Verification items for the finished model (mm, model axes). A direction names the side the tool comes from. Round coordinates to 2 decimals unless told otherwise and drop trailing zeros. Loops run counter-clockwise (first coordinate to the right, second up) from the corner with the lowest first, then second, coordinate; pieces in that order, holes last. Notation, with made-up numbers: (-10.5, -39) - (43.5, -39) arc R29 cw to (43.5, -14) - close; hole circle Ø10 at (-4, 33). An arc over 180 degrees is marked (long way). Use a Markdown table: item, result. Add a question column.
```python
from build123d import *

# Parameters (mm, degrees)
CUT_EXTRUDE_START        = -35
CUT_EXTRUDE_1_DEPTH      = 35
CUT_EXTRUDE_2_DEPTH      = 185.932420089
CUT_EXTRUDE_2_DEPTH_BACK = 185.932420089
SKETCH_4_R               = 7
SKETCH_4_R_2             = 10
SKETCH_5_W               = 35
SKETCH_5_H               = 14
CUT_EXTRUDE_3_DEPTH      = 4
CHAMFER_1_SIZE           = 2


with BuildPart() as part:
    # Эскиз2 → Повернуть1 (revolve)
    with BuildSketch(Plane.XY):
        Polygon((0, 0), (0, 20), (60, 20), (60, 30), (110, 30), (110, 24), (180, 24), (180, 0), align=None)
    revolve(axis=Axis((180, 0, 0), (-1, 0, 0)))

    # Эскиз3 → Вырез-Вытянуть1 (cut)
    with BuildSketch(Plane.ZY.offset(CUT_EXTRUDE_START)):
        with BuildLine():
            Line((-16, 12), (16, 12))
            ThreePointArc((16, 12), (0, 20), (-16, 12))
        make_face()
    extrude(amount=CUT_EXTRUDE_1_DEPTH, mode=Mode.SUBTRACT)

    # Эскиз4 → Вырез-Вытянуть2 (cut, two sides: drawn at the far end of the back side and taken through both)
    with BuildSketch(Plane(origin=(0, 0, 0), x_dir=(1, 0, 0), z_dir=(0, 1, 0)).offset(-CUT_EXTRUDE_2_DEPTH_BACK)):
        with Locations(Location((17.5, 0, 0), (0, 0, 270))):
            Circle(SKETCH_4_R)
        with Locations(Location((85, 0, 0), (0, 0, 270))):
            Circle(SKETCH_4_R_2)
    extrude(amount=CUT_EXTRUDE_2_DEPTH + CUT_EXTRUDE_2_DEPTH_BACK, mode=Mode.SUBTRACT)

    # Эскиз5 → Вырез-Вытянуть3 (cut)
    with BuildSketch(Plane(origin=(0, 24, 0), x_dir=(1, 0, 0), z_dir=(0, 1, 0))):
        with Locations((147.5, 0)):
            Rectangle(SKETCH_5_W, SKETCH_5_H)
    extrude(amount=-CUT_EXTRUDE_3_DEPTH, mode=Mode.SUBTRACT)

    # Фаска1
    chamfer_1_edges = [part.edges().sort_by_distance(p)[0] for p in [
        (180, -24, 0),
        (0, -20, 0),
    ]]
    chamfer(chamfer_1_edges, length=CHAMFER_1_SIZE)


solid = part.part
```
Q1. Section check A-A on y = 0. Record the cut outline in (x, z), plus the area to 3 significant figures.
Q2. Section check B-B on z = 0. State how many separate pieces and enclosed holes the cut face has, plus the area to 3 significant figures.
Q3. Section check D-D on x = 46. Record the cut outline in (y, z), plus the area to 3 significant figures.
Q4. Release check for a two-part mould opening along Z. For faces 1 (the face through (165, 22, 0)), 2 (the face through (94.915, -0.426, -1.302)), 3 (the face through (17.7, 12, -7.3)), 4 (the face through (0.13, -18.12, -0.58)) record: +Z half, -Z half, draft (parallel to the pull), parting line (faces both ways), or undercut.
Q5. Go/stop test with flat-tipped pins: pin 1 Ø3 at (y, z) = (20.5, -17.5) entering from +X; pin 2 Ø7 at (x, z) = (139, -0.5) entering from +Y; pin 3 Ø4 at (x, z) = (129.5, 13.5) entering from +Y. Record where each tip stops, or that it passes through.
Q6. Set-up check for faces 5 (the face through (35, 15, 0)), 6 (the face through (130, 22, 0)), 7 (the face through (110, -13.5, -20.1)): record each of +Z, -Z, +X, -X, +Y, -Y from which the full face is reachable in a straight line by a thin tool's end or side.
Q7. Thickness scan on line 1 along X through (y, z) = (0, 0); line 2 along Z through (x, y) = (85, -1); line 3 along Y through (x, z) = (19, 12). Record the ranges inside material, lowest first.
Q8. Section check C-C on x = 77.5. Record the cut outline in (y, z), plus the area to 3 significant figures.
Determined:
| question | item | result |
|---|---|---|
| 1 | outline | (0, -18) - (2, -20) - (60, -20) - (60, -30) - (110, -30) - (110, -24) - (178, -24) - (180, -22) - (180, 22) - (178, 24) - (110, 24) - (110, 30) - (60, 30) - (60, 20) - (2, 20) - (0, 18) - close; hole circle Ø14 at (17.5, 0); hole circle Ø20 at (85, 0) |
| 1 | area | 8,280 mm² |
| 2 | separate pieces | 3 |
| 2 | enclosed holes | 0 |
| 2 | area | 6,690 mm² |
| 3 | outline | circle Ø40 at (0, 0) |
| 3 | area | 1,260 mm² |
| 4 | face 1 | undercut |
| 4 | face 2 | undercut |
| 4 | face 3 | draft |
| 4 | face 4 | parting line |
| 5 | pin 1 | stops at x = 110 |
| 5 | pin 2 | stops at y = 20 |
| 5 | pin 3 | stops at y = 21.07 |
| 6 | face 5 | +Z, -Z, -X, +Y |
| 6 | face 6 | +Y |
| 6 | face 7 | +X |
| 7 | line 1 | x = 0 to 10.5, 24.5 to 75, 95 to 180 |
| 7 | line 2 | z = -29.98 to -10, 10 to 29.98 |
| 7 | line 3 | y = -16 to 12 |
| 8 | outline | (-29.26, -6.61) arc R30 ccw to (29.26, -6.61) - close; (-29.26, 6.61) - (29.26, 6.61) arc R30 ccw to start |
| 8 | area | 2,040 mm² |
